Could you check a few things on this model? Use its own coordinates, in mm. Round coordinates to 2 decimals unless told otherwise and drop trailing zeros. Write each loop counter-clockwise with the first axis right and the second up, starting at its lowest first coordinate (ties: lowest second). Pieces come first, ordered by that corner, then holes. Notation, with made-up numbers: (83, 11) - (113, 11) arc R20 ccw to (113, 39) - close; hole circle Ø7 at (46, 12). An arc over 180 degrees is marked (long way). Put each result on its own line as item: value.
from build123d import *

# Parameters (mm, degrees)
SKETCH1_R           = 70
SKETCH1_R_2         = 65
SKETCH1_R_3         = 55
BOSS_EXTRUDE1_DEPTH = 5
SKETCH2_R           = 70
SKETCH2_R_2         = 65
BOSS_EXTRUDE2_DEPTH = 20.4
FILLET1_R           = 2.5


with BuildPart() as part:
    # Sketch1 → Boss-Extrude1 (new body)
    # profile 1 of 3: a face of its own
    with BuildSketch(Plane(origin=(0, 0, 0), x_dir=(1, 0, 0), z_dir=(0, 1, 0))):
        with Locations(Location((0, 0, 0), (0, 0, 270))):
            Circle(SKETCH1_R)
        Circle(SKETCH1_R_2, mode=Mode.SUBTRACT)
    # profile 2 of 3: a face of its own
    with BuildSketch(Plane(origin=(0, 0, 0), x_dir=(1, 0, 0), z_dir=(0, 1, 0))):
        Circle(SKETCH1_R_2)
        Circle(SKETCH1_R_3, mode=Mode.SUBTRACT)
    # profile 3 of 3: a face of its own
    with BuildSketch(Plane(origin=(0, 0, 0), x_dir=(1, 0, 0), z_dir=(0, 1, 0))):
        Circle(SKETCH1_R_3)
    extrude(amount=BOSS_EXTRUDE1_DEPTH)

    # Sketch2 → Boss-Extrude2 (add)
    with BuildSketch(Plane(origin=(0, 5, 0), x_dir=(1, 0, 0), z_dir=(0, 1, 0))):
        with Locations(Location((0, 0, 0), (0, 0, 270))):
            Circle(SKETCH2_R)
        with Locations(Location((0, 0, 0), (0, 0, 270))):
            Circle(SKETCH2_R_2, mode=Mode.SUBTRACT)
    extrude(amount=BOSS_EXTRUDE2_DEPTH)

    # Fillet1
    fillet1_edges = [part.edges().sort_by_distance(p)[0] for p in [
        (0, 5, -65),
    ]]
    fillet(fillet1_edges, radius=FILLET1_R)


solid = part.part
(1) I'm going to push flat-ended pins straight in: pin 1 (1.5 mm diameter, centred on x = -33.5, y = 10, fed in from -Z); pin 2 (4 mm diameter, centred on y = 8, z = 1, fed in from +X); pin 3 (8 mm diameter, centred on x = -17, y = 3, fed in from -Z). Where does each tip first touch, or does it pass through?
Values found:
pin 1: stops at z = -61.87
pin 2: stops at x = 70
pin 3: stops at z = -68.78
(2) Imagine slicing it at A-A, the plane z = 0. List the corners of the cut face in (x, y) for me, then the cut area to 3 significant figures.
Values found:
outline: (-70, 0) - (70, 0) - (70, 25.4) - (65, 25.4) - (65, 7.5) arc R2.5 cw to (62.5, 5) - (-62.5, 5) arc R2.5 cw to (-65, 7.5) - (-65, 25.4) - (-70, 25.4) - close
area: 907 mm^2
(3) If we mould it in two halves opening along Z, with no side actions, what happens to faces 1 (the face through (19.52, 16.32, 62)), 2 (the face through (1, 5, -1)), 3 (the face through (-42.594, 12.522, -55.55)), 4 (the face through (-1, 0, -1))? For each: pulls with the +Z half, pulls with the -Z half, needs draft (parallel to the pull), parting line crosses it, or undercut.
Values found:
face 1: undercut
face 2: undercut
face 3: parting line crosses it
face 4: needs draft
(4) Imagine slicing it at B-B, the plane x = 0. List the corners of the cut face in (y, z) for me.
Values found:
outline: (0, -70) - (25.4, -70) - (25.4, -65) - (7.5, -65) arc R2.5 cw to (5, -62.5) - (5, 62.5) arc R2.5 cw to (7.5, 65) - (25.4, 65) - (25.4, 70) - (0, 70) - close
(5) Please list where these lines run through material, in increasing order: probe 1 along X at (y, z) = (13.75, 0); probe 2 along Y at (x, z) = (24.5, 6); probe 3 along X at (y, z) = (15, 39.5). Write a range as from..to.
Values found:
probe 1: x = -70..-65, 65..70
probe 2: y = 0..5
probe 3: x = -57.79..-51.62, 51.62..57.79
(6) Imagine slicing it at C-C, the plane y = 15.5. List the corners of the cut face in (x, z) for me.
Values found:
outline: circle Ø140 at (0, 0); hole circle Ø130 at (0, 0)
